from build123d import *

# Parameters (mm, degrees)
SKETCH_1_W          = 24.73
SKETCH_1_H          = 45.23
EXTRUDE_1_DEPTH     = 32
CHAMFER_1_SIZE      = 2
EXTRUDE_2_DEPTH     = 1
SKETCH_3_R          = 1
CUT_EXTRUDE_1_DEPTH = 4
SKETCH_4_R          = 9.975
EXTRUDE_3_DEPTH     = 2
SKETCH_5_R          = 2
SKETCH_5_R_2        = 1
CUT_EXTRUDE_2_DEPTH = 3
SKETCH_6_W          = 20.33
SKETCH_6_H          = 12
EXTRUDE_4_DEPTH     = 2
CHAMFER_2_SIZE      = 2
SKETCH_7_W          = 22.33
SKETCH_7_H          = 5
CUT_EXTRUDE_3_DEPTH = 2
SKETCH_8_R          = 3
EXTRUDE_5_DEPTH     = 4.1
CUT_EXTRUDE_START   = -4
SKETCH_9_R          = 1
CUT_EXTRUDE_4_DEPTH = 4
FILLET_1_R          = 1


with BuildPart() as part:
    # 스케치1 → 보스-돌출1 (new body)
    with BuildSketch(Plane.XY):
        Rectangle(SKETCH_1_W, SKETCH_1_H)
    extrude(amount=EXTRUDE_1_DEPTH)

    # 모따기1
    chamfer_1_edges = [part.edges().sort_by_distance(p)[0] for p in [
        (-12.365, 22.615, 16),
        (12.365, 22.615, 16),
    ]]
    chamfer(chamfer_1_edges, length=CHAMFER_1_SIZE)

    # 스케치2 → 보스-돌출2 (add)
    with BuildSketch(Plane.XY.offset(32)):
        with BuildLine():
            Line((-7, -22.615), (7, -22.615))
            Line((7, -22.615), (7, 2.753205655))
            ThreePointArc((7, 2.753205655), (0, 0.5), (-7, 2.753205655))
            Line((-7, 2.753205655), (-7, -22.615))
        make_face()
    extrude(amount=EXTRUDE_2_DEPTH)

    # 스케치3 → 컷-돌출1 (cut)
    with BuildSketch(Plane.XY.offset(32)):
        with Locations((-10.25, 3.885)):
            Circle(SKETCH_3_R)
        with Locations((-10.25, -16.615)):
            Circle(SKETCH_3_R)
        with Locations((10.25, -16.615)):
            Circle(SKETCH_3_R)
        with Locations((10.25, 3.885)):
            Circle(SKETCH_3_R)
    extrude(amount=-CUT_EXTRUDE_1_DEPTH, mode=Mode.SUBTRACT)

    # 스케치4 → 보스-돌출3 (add)
    with BuildSketch(Plane.XY.offset(32)):
        with Locations((0, 12.5)):
            Circle(SKETCH_4_R)
    extrude(amount=EXTRUDE_3_DEPTH)

    # 스케치5 → 컷-돌출2 (cut)
    with BuildSketch(Plane.XY.offset(34)):
        with Locations((0, 12.5)):
            Circle(SKETCH_5_R)
        with Locations((0, 19.5)):
            Circle(SKETCH_5_R_2)
        with Locations((7, 12.5)):
            Circle(SKETCH_5_R_2)
        with Locations((0, 5.5)):
            Circle(SKETCH_5_R_2)
        with Locations((-7, 12.5)):
            Circle(SKETCH_5_R_2)
    extrude(amount=-CUT_EXTRUDE_2_DEPTH, mode=Mode.SUBTRACT)

    # 스케치6 → 보스-돌출4 (add)
    with BuildSketch(Plane(origin=(0, 0, 0), x_dir=(-1, 0, 0), z_dir=(0, 0, -1))):
        with Locations((0, -12.115)):
            Rectangle(SKETCH_6_W, SKETCH_6_H)
    extrude(amount=EXTRUDE_4_DEPTH)

    # 모따기2
    chamfer_2_edges = [part.edges().sort_by_distance(p)[0] for p in [
        (0, -6.115, -2),
    ]]
    chamfer(chamfer_2_edges, length=CHAMFER_2_SIZE - 0.0001)  # a hair under: the kernel refuses the full size

    # 스케치7 → 컷-돌출3 (cut)
    with BuildSketch(Plane(origin=(0, 0, 0), x_dir=(-1, 0, 0), z_dir=(0, 0, -1))):
        with Locations((0, -3.615)):
            Rectangle(SKETCH_7_W, SKETCH_7_H)
    extrude(amount=-CUT_EXTRUDE_3_DEPTH, mode=Mode.SUBTRACT)

    # 스케치8 → 보스-돌출5 (add)
    with BuildSketch(Plane(origin=(0, 0, 0), x_dir=(-1, 0, 0), z_dir=(0, 0, -1))):
        with Locations(Location((0, 12.5, 0), (0, 0, 180))):
            Circle(SKETCH_8_R)
    extrude(amount=EXTRUDE_5_DEPTH)

    # 스케치9 → 컷-돌출4 (cut)
    with BuildSketch(Plane(origin=(0, 0, 0), x_dir=(-1, 0, 0), z_dir=(0, 0, -1)).offset(CUT_EXTRUDE_START)):
        with Locations(Location((-10.25, 3.885, 0), (0, 0, 180))):
            Circle(SKETCH_9_R)
        with Locations(Location((10.25, 3.885, 0), (0, 0, 180))):
            Circle(SKETCH_9_R)
        with Locations((-10.25, -20.615)):
            Circle(SKETCH_9_R)
        with Locations((10.25, -20.615)):
            Circle(SKETCH_9_R)
    extrude(amount=CUT_EXTRUDE_4_DEPTH, mode=Mode.SUBTRACT)

    # 필렛1
    fillet_1_edges = [part.edges().sort_by_distance(p)[0] for p in [
        (12.365, -22.615, 16),
        (-12.365, -22.615, 16),
    ]]
    fillet(fillet_1_edges, radius=FILLET_1_R)


solid = part.part
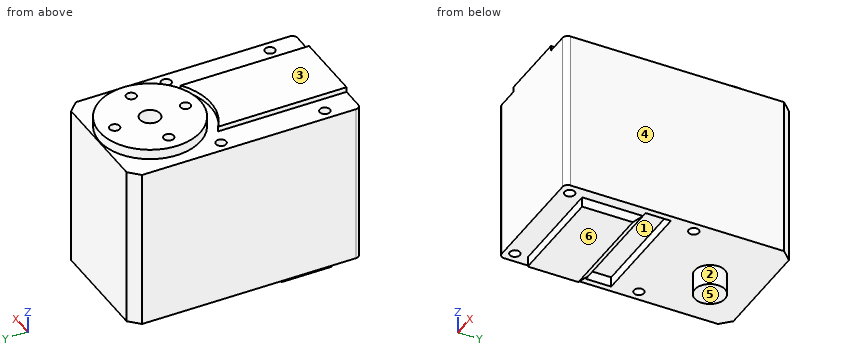
Work out the finished part from the listing and answer in its coordinate system (mm). Face numbers are marked on the shaded views. A direction names the side the tool comes from. Round coordinates to 2 decimals unless told otherwise and drop trailing zeros. Loops run counter-clockwise (first coordinate to the right, second up) from the corner with the lowest first, then second, coordinate; pieces in that order, holes last. Notation, with made-up numbers: M 54.25,2.25 L 109.25,2.25 A22 ccw 109.25,25.25 Z; hole C -25,25.5 d8. An arc over 180 degrees is marked long. One line per question, with ' | ' between items. Start each with the question number.
(1) For a pull along X with two mould halves and no side action, classify the marked faces 1, 2, 3 and 4 as released by +X, released by -X, zero draft, split by the parting line, or undercut.
(2) A tool of negligible diameter and unlimited length cuts with its end or side. For the marked faces 5 and 6, from which of +Z, -Z, +X, -X, +Y, -Y can it reach the whole face along a straight path? Write none if from no direction.
(3) Find the intervals of material crossed by line 1 (Y direction, x = -10.25, z = 1.1) (3 decimals); line 2 (Y direction, x = 0, z = 32.6) (3 decimals); line 3 (Y direction, x = 10.25, z = 2.4) (3 decimals), in increasing order.
(4) A cutting plane is placed at C-C on x = -4.5. Write down the section's boundary in (y, z) (3 decimals).
(5) A cutting plane is placed at D-D on y = 19.5. Write down the section's boundary in (x, z) (3 decimals), plus the area to 3 significant figures.
(6) A cutting plane is placed at A-A on y = -9. Write down the section's boundary in (x, z) (3 decimals).
(7) Flat-ended cylindrical pins translate along their axes: pin 1 Ø1.2 at (x, y) = (10.25, -16.615) entering from +Z; pin 2 Ø1.6 at (y, z) = (-12.5, -0.5) entering from +X (3 decimals); pin 3 Ø1.2 at (x, y) = (10.25, -20.615) entering from -Z; pin 4 Ø1.6 at (y, z) = (-9.5, -1) entering from -X (3 decimals). Find the tip coordinate at first contact, or state that the pin passes through.
Geometry check:
1) face 1: undercut | face 2: split by the parting line | face 3: zero draft | face 4: released by +X
2) face 5: -Z, +X, -X, +Y, -Y | face 6: -Z, +X, -X, -Y
3) line 1: y = -22.615 to -21.615, -19.615 to -6.115, -1.115 to 2.885, 4.885 to 22.615 | line 2: y = -22.615 to 0.5, 2.525 to 4.5, 6.5 to 10.5, 14.5 to 18.5, 20.5 to 22.475 | line 3: y = -22.615 to -21.615, -19.615 to 2.885, 4.885 to 22.615
4) outline: M -22.615,0 L -18.115,0 L -18.115,-2 L -8.115,-2 L -6.115,0 L -6.115,2 L -1.115,2 L -1.115,0 L 22.615,0 L 22.615,32 L 21.402,32 L 21.402,34 L 3.598,34 L 3.598,32 L 1.376,32 L 1.376,33 L -22.615,33 Z
5) outline: M -12.365,0 L 12.365,0 L 12.365,32 L 7.106,32 L 7.106,34 L 1,34 L 1,31 L -1,31 L -1,34 L -7.106,34 L -7.106,32 L -12.365,32 Z | area: 814 mm²
6) outline: M -12.365,0 L -10.165,0 L -10.165,-2 L 10.165,-2 L 10.165,0 L 12.365,0 L 12.365,32 L 7,32 L 7,33 L -7,33 L -7,32 L -12.365,32 Z
7) pin 1: stops at z = 28 | pin 2: stops at x = 12.365 | pin 3: stops at z = 4 | pin 4: stops at x = -10.165
